Geometry: final body of the model. Coordinates: model frame, mm. Coordinates: 2 decimals unless noted, no trailing zeros. Order: outer loops, then holes, each group sorted by start corner. A loop starts at its lowest first (then second) coordinate and runs counter-clockwise, first axis right, second up. Notation, with made-up numbers: (43.25, 31.5) -> (65.25, 31.5) arc R29 cw to (65.25, 60.5) -> close; hole circle Ø2 at (-10, -18). An arc over 180 degrees is marked (long way). Use CSV: the item, a comma, the result in double quotes. Start each with the question number.
from build123d import *

# Parameters (mm, degrees)
PAD014_DEPTH         = 3
SKETCH055_R          = 1.7
POCKET019_DEPTH      = 363.445695
POCKET019_DEPTH_BACK = 366.445695


with BuildPart() as part:
    # Sketch052 → Pad014 (new body)
    with BuildSketch(Plane.XY):
        with BuildLine():
            ThreePointArc((152.862483, 128.734095), (84.297377, 181.199774), (0, 199.848457))
            Line((0, 199.848457), (0, 209.848457))
            ThreePointArc((160.511403, 135.17568), (88.515442, 190.266633), (0, 209.848457))
            ThreePointArc((152.862483, 128.734095), (159.907736, 128.130427), (160.511403, 135.17568))
        make_face()
    pad014 = extrude(amount=PAD014_DEPTH)

    # Sketch055 → Pocket019 (cut, two sides)
    with BuildSketch(Plane.XY) as pocket019_sk:
        with Locations((143.11, 146.568818)):
            Circle(SKETCH055_R)
        with BuildLine():
            Line((0, 203.148457), (0, 206.548457))
            ThreePointArc((0, 203.148457), (1.7, 204.848457), (0, 206.548457))
        make_face()
    pocket019 = extrude(amount=-POCKET019_DEPTH, mode=Mode.SUBTRACT) + extrude(pocket019_sk.sketch, amount=POCKET019_DEPTH_BACK, mode=Mode.SUBTRACT)

    # Mirrored019: Pad014, Pocket019 across Sketch052 V_Axis
    add(pad014.mirror(Plane(origin=(0, 0, 0), x_dir=(0, 0, 1), z_dir=(1, 0, 0))))
    add(pocket019.mirror(Plane(origin=(0, 0, 0), x_dir=(0, 0, 1), z_dir=(1, 0, 0))), mode=Mode.SUBTRACT)


solid = part.part
(1) Section B-B (z = 0.65). Return loops of the section in (x, y).
(2) Section A-A (y = 172). Return loops of the section in (x, z).
(3) First-contact query: pin 1 (4 mm diameter, centred on x = 113, y = 167, fed in from -Z); pin 2 (1.5 mm diameter, centred on y = 182, z = 2.5, fed in from -X); pin 3 (1.5 mm diameter, centred on x = -99.5, z = 1.5, fed in from -Y). Flat tips, straight axial feed; report the tip coordinate or a pass-through.
(4) Section D-D (x = -7). Return loops of the section in (y, z).
(5) Section C-C (x = 75). Return loops of the section in (y, z), then the cut area to 3 significant figures.
(6) Line query: line 1 (X direction, y = 134.5, z = 2.75); line 2 (Y direction, x = 0, z = 0.95); line 3 (X direction, y = 161.5, z = 2.35). Output: solid intervals per line, ascending. Write a range as from..to.
Check sheet entries:
1,outline,"(-160.51, 135.18) arc R5 ccw to (-152.86, 128.73) arc R199.85 cw to (0, 199.85) arc R199.85 cw to (152.86, 128.73) arc R5 ccw to (160.51, 135.18) arc R209.85 ccw to (0, 209.85) arc R209.85 ccw to start; hole circle Ø3.4 at (-143.11, 146.57); hole circle Ø3.4 at (0, 204.85); hole circle Ø3.4 at (143.11, 146.57)"
2,outline,"(-120.22, 0) -> (-101.76, 0) -> (-101.76, 3) -> (-120.22, 3) -> close; (101.76, 0) -> (120.22, 0) -> (120.22, 3) -> (101.76, 3) -> close"
3,pin 1,"stops at z = 0"
3,pin 2,"stops at x = -105.76"
3,pin 3,"stops at y = 172.89"
4,outline,"(199.73, 0) -> (209.73, 0) -> (209.73, 3) -> (199.73, 3) -> close"
5,outline,"(185.24, 0) -> (195.99, 0) -> (195.99, 3) -> (185.24, 3) -> close"
5,area,"32.2 mm^2"
6,line 1,"x = -160.99..-147.81, 147.81..160.99"
6,line 2,"y = 199.85..203.15, 206.55..209.85"
6,line 3,"x = -133.99..-117.72, 117.72..133.99"
